Read the model definition and answer for the solid it produces. Units are mm, in the model's axes. A direction names the side the tool comes from. Coordinates: 2 decimals unless noted, no trailing zeros. Loops run counter-clockwise (first coordinate to the right, second up) from the corner with the lowest first, then second, coordinate; pieces in that order, holes last. Notation, with made-up numbers: (18, -37) -> (35, -37) arc R23 cw to (35, -17) -> close; hole circle Ø9 at (34.25, 64). An arc over 180 degrees is marked (long way). Answer in a Markdown table with one row per item.
```python
from build123d import *

# Parameters (mm, degrees)
BOSS_EXTRUDE1_DEPTH = 3.175
SKETCH2_R           = 1.6
CUT_EXTRUDE1_DEPTH  = 164.054057029
SKETCH3_R           = 5
SKETCH3_R_2         = 1.6
SKETCH3_R_3         = 5.5
CUT_EXTRUDE2_DEPTH  = 164.054057029
SKETCH5_R           = 1.524
CUT_EXTRUDE3_DEPTH  = 164.054057029
CUT_EXTRUDE4_DEPTH  = 164.054057029
SKETCH8_R           = 1.25
CUT_EXTRUDE5_DEPTH  = 164.054057029
SKETCH9_W           = 27.941695013
SKETCH9_H           = 13.477758771
SKETCH9_W_2         = 30.242775778
SKETCH9_H_2         = 17.203318106
SKETCH9_W_3         = 23.480845259
SKETCH9_H_3         = 15.425198082
SKETCH9_W_4         = 27.275197361
SKETCH9_H_4         = 16.833910872
BOSS_EXTRUDE2_DEPTH = 3.175
SKETCH16_R          = 1.6
CUT_EXTRUDE6_DEPTH  = 10
FILLET1_R           = 3
FILLET2_R           = 1


with BuildPart() as part:
    # Sketch1 → Boss-Extrude1 (new body)
    with BuildSketch(Plane(origin=(0, 0, 0), x_dir=(1, 0, 0), z_dir=(0, 1, 0))):
        Polygon((115.274769331, 0), (81.511571094, 81.511571094), (0, 115.274769331), (-81.511571094, 81.511571094), (-115.274769331, 0), (-81.511571094, -81.511571094), (0, -115.274769331), (81.511571094, -81.511571094), align=None)
    extrude(amount=BOSS_EXTRUDE1_DEPTH)

    # Sketch2 → Cut-Extrude1 (cut, through all)
    with BuildSketch(Plane(origin=(0, 3.175, 0), x_dir=(1, 0, 0), z_dir=(0, 1, 0))):
        with Locations(Location((-8.982761909, 81.788202013, 0), (0, 0, 270))):
            Circle(SKETCH2_R)
        with Locations(Location((3.951551546, 87.145770066, 0), (0, 0, 270))):
            Circle(SKETCH2_R)
        with Locations(Location((-64.41553386, 58.827196071, 0), (0, 0, 90))):
            Circle(SKETCH2_R)
        with Locations(Location((-51.481220405, 64.184764124, 0), (0, 0, 90))):
            Circle(SKETCH2_R)
        with Locations(Location((64.41553386, -58.827196071, 0), (0, 0, 90))):
            Circle(SKETCH2_R)
        with Locations(Location((51.481220405, -64.184764124, 0), (0, 0, 90))):
            Circle(SKETCH2_R)
        with Locations(Location((8.982761909, -81.788202013, 0), (0, 0, 270))):
            Circle(SKETCH2_R)
        with Locations(Location((-3.951551546, -87.145770066, 0), (0, 0, 270))):
            Circle(SKETCH2_R)
    extrude(amount=-CUT_EXTRUDE1_DEPTH, mode=Mode.SUBTRACT)

    # Sketch3 → Cut-Extrude2 (cut, through all)
    with BuildSketch(Plane(origin=(0, 3.175, 0), x_dir=(1, 0, 0), z_dir=(0, 1, 0))):
        with Locations(Location((-96.010047769, 20.377892773, 0), (0, 0, 270))):
            Circle(SKETCH3_R)
        with Locations(Location((20.377892773, -96.010047769, 0), (0, 0, 270))):
            Circle(SKETCH3_R_2)
        with Locations(Location((53.480009673, -82.298702006, 0), (0, 0, 90))):
            Circle(SKETCH3_R_2)
        with Locations(Location((-24.491739671, 86.844676056, 0), (0, 0, 270))):
            Circle(SKETCH3_R_2)
        with Locations(Location((-44.090184145, 78.726734554, 0), (0, 0, 90))):
            Circle(SKETCH3_R_2)
        with Locations(Location((-35.972242642, 59.128290081, 0), (0, 0, 270))):
            Circle(SKETCH3_R_2)
        with Locations(Location((-16.373798169, 67.246231583, 0), (0, 0, 90))):
            Circle(SKETCH3_R_2)
        with Locations(Location((53.480009673, 82.298702006, 0), (0, 0, 270))):
            Circle(SKETCH3_R_3)
        Polygon((-68.117650961, -70.823631462), (-71.944485285, -80.062426787), (-51.944485285, -88.346698034), (-48.117650961, -79.107902709), align=None)
        Polygon((-1.913417162, -98.246322988), (-5.740251485, -107.485118313), (-25.740251485, -99.200847065), (-21.913417162, -89.96205174), align=None)
        Polygon((88.346698034, -51.944485285), (80.062426787, -71.944485285), (70.823631462, -68.117650961), (79.107902709, -48.117650961), align=None)
        Polygon((98.246322988, -1.913417162), (107.485118313, -5.740251485), (99.200847066, -25.740251485), (89.96205174, -21.913417162), align=None)
    extrude(amount=-CUT_EXTRUDE2_DEPTH, mode=Mode.SUBTRACT)

    # Sketch5 → Cut-Extrude3 (cut, through all)
    with BuildSketch(Plane(origin=(0, 3.175, 0), x_dir=(1, 0, 0), z_dir=(0, 1, 0))):
        with Locations(Location((33.228392199, -17.165706419, 0), (0, 0, 270))):
            Circle(SKETCH5_R)
        with Locations(Location((-11.35803404, -35.634008864, 0), (0, 0, 270))):
            Circle(SKETCH5_R)
        with Locations(Location((-33.697130397, 26.59401536, 0), (0, 0, 270))):
            Circle(SKETCH5_R)
        with Locations(Location((5.02266081, 42.632278011, 0), (0, 0, 270))):
            Circle(SKETCH5_R)
    extrude(amount=-CUT_EXTRUDE3_DEPTH, mode=Mode.SUBTRACT)

    # Sketch6 → Cut-Extrude4 (cut, through all)
    with BuildSketch(Plane(origin=(0, 3.175, 0), x_dir=(1, 0, 0), z_dir=(0, 1, 0))):
        Polygon((41.137502582, -7.855309115), (23.534064693, 34.643149381), (-41.137502582, 7.855309115), (-23.534064693, -34.643149381), align=None)
    extrude(amount=-CUT_EXTRUDE4_DEPTH, mode=Mode.SUBTRACT)

    # Sketch8 → Cut-Extrude5 (cut, through all)
    with BuildSketch(Plane(origin=(0, 3.175, 0), x_dir=(1, 0, 0), z_dir=(0, 1, 0))):
        with Locations(Location((-55.208521245, -56.963472567, 0), (0, 0, 270))):
            Circle(SKETCH8_R)
        with Locations(Location((-26.106315971, -44.908944448, 0), (0, 0, 270))):
            Circle(SKETCH8_R)
        with Locations(Location((-84.675145537, 14.175251436, 0), (0, 0, 270))):
            Circle(SKETCH8_R)
        with Locations(Location((-55.572940263, 26.229779555, 0), (0, 0, 270))):
            Circle(SKETCH8_R)
    extrude(amount=-CUT_EXTRUDE5_DEPTH, mode=Mode.SUBTRACT)

    # Sketch9 → Boss-Extrude2 (add)
    with BuildSketch(Plane(origin=(0, 3.175, 0), x_dir=(1, 0, 0), z_dir=(0, 1, 0))):
        with Locations((-58.48921623, 61.487322726)):
            Rectangle(SKETCH9_W, SKETCH9_H)
        with Locations((3.475601533, 82.74492599)):
            Rectangle(SKETCH9_W_2, SKETCH9_H_2)
        with Locations((2.615763969, -84.269263782)):
            Rectangle(SKETCH9_W_3, SKETCH9_H_3)
        with Locations((52.818476628, -60.231828394)):
            Rectangle(SKETCH9_W_4, SKETCH9_H_4)
    extrude(amount=-BOSS_EXTRUDE2_DEPTH)

    # Sketch16 → Cut-Extrude6 (cut)
    with BuildSketch(Plane(origin=(0, 3.175, 0), x_dir=(1, 0, 0), z_dir=(0, 1, 0))):
        with Locations(Location((-51.719028062, 64.497570003, 0), (0, 0, 270))):
            Circle(SKETCH16_R)
        with Locations(Location((-63.082746312, 59.790563785, 0), (0, 0, 270))):
            Circle(SKETCH16_R)
        with Locations(Location((-9.03579366, 82.177544578, 0), (0, 0, 270))):
            Circle(SKETCH16_R)
        with Locations(Location((2.32792459, 86.884550796, 0), (0, 0, 270))):
            Circle(SKETCH16_R)
        with Locations(Location((63.082746312, -59.790563785, 0), (0, 0, 270))):
            Circle(SKETCH16_R)
        with Locations(Location((51.719028062, -64.497570003, 0), (0, 0, 270))):
            Circle(SKETCH16_R)
        with Locations(Location((9.03579366, -82.177544578, 0), (0, 0, 270))):
            Circle(SKETCH16_R)
        with Locations(Location((-2.32792459, -86.884550796, 0), (0, 0, 270))):
            Circle(SKETCH16_R)
    extrude(amount=-CUT_EXTRUDE6_DEPTH, mode=Mode.SUBTRACT)

    # Fillet1
    fillet1_edges = [part.edges().sort_by_distance(p)[0] for p in [
        (81.511571094, 1.5875, 81.511571094),
        (0, 1.5875, 115.274769331),
        (-81.511571094, 1.5875, 81.511571094),
        (-115.274769331, 1.5875, 0),
        (-81.511571094, 1.5875, -81.511571094),
        (0, 1.5875, -115.274769331),
        (81.511571094, 1.5875, -81.511571094),
        (115.274769331, 1.5875, 0),
    ]]
    fillet(fillet1_edges, radius=FILLET1_R)

    # Fillet2
    fillet2_edges = [part.edges().sort_by_distance(p)[0] for p in [
        (79.107902709, 1.5875, 48.117650961),
        (88.346698034, 1.5875, 51.944485285),
        (80.062426787, 1.5875, 71.944485285),
        (70.823631462, 1.5875, 68.117650961),
        (89.96205174, 1.5875, 21.913417162),
        (98.246322988, 1.5875, 1.913417162),
        (107.485118313, 1.5875, 5.740251485),
        (99.200847066, 1.5875, 25.740251485),
        (-51.944485285, 1.5875, 88.346698034),
        (-71.944485285, 1.5875, 80.062426787),
        (-68.117650961, 1.5875, 70.823631462),
        (-48.117650961, 1.5875, 79.107902709),
        (-21.913417162, 1.5875, 89.96205174),
        (-1.913417162, 1.5875, 98.246322988),
        (-5.740251485, 1.5875, 107.485118313),
        (-25.740251485, 1.5875, 99.200847065),
    ]]
    fillet(fillet2_edges, radius=FILLET2_R)


solid = part.part
```
1. A cutting plane is placed at B-B on y = 1.55. Count the separate pieces of the cut face and the enclosed holes in it, and give its area (3 significant figures).
A:
| item | result |
|---|---|
| separate pieces | 1 |
| enclosed holes | 29 |
| area | 33,200 mm2 |
2. Find the intervals of material crossed by probe 1 along X at (y, z) = (2, -25.5); probe 2 along X at (y, z) = (2.8, -27); probe 3 along Z at (x, y) = (8, 1.75), in increasing order.
A:
| item | result |
|---|---|
| probe 1 | x = -104.71 to -56.59, -54.56 to -34.76, -32.64 to 1.46, 27.32 to 104.71 |
| probe 2 | x = -104.09 to -56.56, -54.59 to -35.17, -32.23 to 5.08, 26.7 to 104.09 |
| probe 3 | z = -111.96 to -28.21, 21.58 to 80.96, 83.4 to 111.96 |
3. A cutting plane is placed at A-A on z = 11. Give the vertices of the cut face in (x, y) (3 decimals), and give its area (3 significant figures).
A:
| item | result |
|---|---|
| outline | (-110.718, 0) -> (-33.327, 0) -> (-33.327, 3.175) -> (-110.718, 3.175) -> close; (33.546, 0) -> (94.483, 0) -> (94.483, 3.175) -> (33.546, 3.175) -> close; (105.306, 0) -> (110.718, 0) -> (110.718, 3.175) -> (105.306, 3.175) -> close |
| area | 456 mm2 |
4. Given pin 1 Ø1.5 at (x, z) = (-26.11, 44.91) entering from -Y; pin 2 Ø1 at (x, y) = (6, 2.5) entering from +Z, each flat-ended and moving along its own axis, determine where each tip first touches the part or whether it passes through.
A:
| item | result |
|---|---|
| pin 1 | passes through |
| pin 2 | stops at z = 113 |
5. A tool of negligible diameter and unlimited length cuts with its end or side. For faces 1 (the flat face through (-2, 3.175, -27)), 2 (the flat face through (-8.349, 1.61, -21.437)), from which of +Z, -Z, +X, -X, +Y, -Y can it reach the whole face along a straight path? Write none if from no direction.
A:
| item | result |
|---|---|
| face 1 | +Z, -Z, +X, -X, +Y |
| face 2 | +Y, -Y |
6. The mould has two halves that part along Z. Classify faces 3 (the flat face through (98.623, 1.565, -40.201)), 4 (the flat face through (98.163, 1.565, 41.31)), 5 (the flat face through (-15.6, 1.6, 103.4)): pulls with the +Z half, pulls with the -Z half, needs draft (parallel to the pull), parting line crosses it, or undercut.
A:
| item | result |
|---|---|
| face 3 | pulls with the -Z half |
| face 4 | pulls with the +Z half |
| face 5 | undercut |
